Geometry check sheet. Reference: the model listing, model coordinates, mm. Face numbers are marked on the shaded views. A direction names the side the tool comes from. Give positions to 0.01 mm unless a question says otherwise; leave off trailing zeros. Order: outer loops, then holes, each group sorted by start corner. A loop starts at its lowest first (then second) coordinate and runs counter-clockwise, first axis right, second up. Notation, with made-up numbers: M 38.5,82 L 77.5,82 A5 ccw 77.5,86 Z; hole C -7.5,20.5 d11. An arc over 180 degrees is marked long. Answer as CSV lines item,"result".
from build123d import *

# Parameters (mm, degrees)
SKETCH7_R               = 2.5
CUT_EXTRUDE2_DEPTH      = 4
CUT_EXTRUDE3_DEPTH      = 4
CUT_EXTRUDE3_DEPTH_BACK = 4
SKETCH8_W               = 2.5
SKETCH8_H               = 7.259020633
FILLET1_R               = 1.5
SKETCH9_W               = 2.5
SKETCH9_H               = 5.356071321
CUT_EXTRUDE4_DEPTH      = 10
FILLET2_R               = 1.25
SKETCH10_W              = 2.503236591
SKETCH10_H              = 5.356071321
CUT_EXTRUDE5_DEPTH      = 10
SKETCH11_W              = 2.503236591
SKETCH11_H              = 6.001405943
CUT_EXTRUDE6_DEPTH      = 10
FILLET4_R               = 1.25
SKETCH12_W              = 2.514787158
SKETCH12_H              = 5.75
CUT_EXTRUDE9_DEPTH      = 10
SKETCH14_R              = 1.249039751
CUT_EXTRUDE10_DEPTH     = 10


# Some blends are built 0.0001 mm under size
with BuildPart() as part:
    # Sketch5 → Revolve3 (revolve)
    with BuildSketch(Plane.XY, mode=Mode.PRIVATE) as revolve3_sk:
        Polygon((0, 0), (5.5, 0), (5.5, 1), (7, 1), (7, 3), (3, 6), (0, 6), align=None)
    revolve(revolve3_sk.sketch.rotate(Axis((0, 6, 0), (0, -1, 0)), 180), axis=Axis((0, 6, 0), (0, -1, 0)))

    # Sketch7 → Cut-Extrude2 (cut)
    with BuildSketch(Plane(origin=(0, 6, 0), x_dir=(1, 0, 0), z_dir=(0, 1, 0))):
        with Locations(Location((0, 0, 0), (0, 0, 180))):
            Circle(SKETCH7_R)
    extrude(amount=-CUT_EXTRUDE2_DEPTH, mode=Mode.SUBTRACT)

    # Sketch8 → Cut-Extrude3 (cut, two sides: drawn at the far end of the back side and taken through both)
    with BuildSketch(Plane(origin=(0, 2, 0), x_dir=(1, 0, 0), z_dir=(0, 1, 0)).offset(-CUT_EXTRUDE3_DEPTH_BACK)):
        with Locations((0, -3.629510317)):
            Rectangle(SKETCH8_W, SKETCH8_H)
    extrude(amount=CUT_EXTRUDE3_DEPTH + CUT_EXTRUDE3_DEPTH_BACK, mode=Mode.SUBTRACT)

    # Fillet1
    # the kernel refuses this fillet: 1.5 mm, written as the material it adds along each edge
    with BuildSketch(Plane(origin=(1.25, 2, 0), x_dir=(-1, 0, 0), z_dir=(0, -1, 0)), Plane(origin=(-1.25, 0, 0), x_dir=(1, 0, 0), z_dir=(0, 1, 0))) as fillet1_piece_1:
        with BuildLine():
            CenterArc((FILLET1_R, -FILLET1_R), FILLET1_R, 90, 90)
            Line((0, -FILLET1_R), (0, 0))
            Line((0, 0), (FILLET1_R, 0))
        make_face()
    extrude(amount=2)

    # Sketch9 → Cut-Extrude4 (cut)
    with BuildSketch(Plane(origin=(0, 0, 0), x_dir=(-1, 0, 0), z_dir=(0, -1, 0))):
        with Locations((0, -2.67803566)):
            Rectangle(SKETCH9_W, SKETCH9_H)
    extrude(amount=-CUT_EXTRUDE4_DEPTH, mode=Mode.SUBTRACT)

    # Fillet2
    fillet2_edges = [part.edges().sort_by_distance(p)[0] for p in [
        (-1.25, 1, 0),
        (1.25, 1, 0),
    ]]
    fillet(fillet2_edges, radius=FILLET2_R - 0.0001)  # a hair under: the kernel refuses the full size

    # Sketch10 → Cut-Extrude5 (cut)
    with BuildSketch(Plane.XZ):
        with Locations((-0.001618296, 2.67803566)):
            Rectangle(SKETCH10_W, SKETCH10_H)
    extrude(amount=-CUT_EXTRUDE5_DEPTH, mode=Mode.SUBTRACT)

    # Sketch11 → Cut-Extrude6 (cut)
    with BuildSketch(Plane(origin=(0, 0, 0), x_dir=(-1, 0, 0), z_dir=(0, -1, 0))):
        with Locations((0.001618296, -2.355368349)):
            Rectangle(SKETCH11_W, SKETCH11_H)
    extrude(amount=-CUT_EXTRUDE6_DEPTH, mode=Mode.SUBTRACT)

    # Fillet4
    fillet4_edges = [part.edges().sort_by_distance(p)[0] for p in [
        (1.25, 1, -0.645334622),
        (-1.253236591, 1, -0.645334622),
    ]]
    fillet(fillet4_edges, radius=FILLET4_R)

    # Sketch12 → Cut-Extrude9 (cut)
    with BuildSketch(Plane.XZ):
        with Locations((-0.007393579, 2.481071321)):
            Rectangle(SKETCH12_W, SKETCH12_H)
    extrude(amount=-CUT_EXTRUDE9_DEPTH, mode=Mode.SUBTRACT)

    # Sketch14 → Cut-Extrude10 (cut)
    with BuildSketch(Plane(origin=(0, 0, 0), x_dir=(-1, 0, 0), z_dir=(0, -1, 0))):
        with Locations((0.007393579, 0.393928679)):
            Circle(SKETCH14_R)
    extrude(amount=-CUT_EXTRUDE10_DEPTH, mode=Mode.SUBTRACT)


solid = part.part
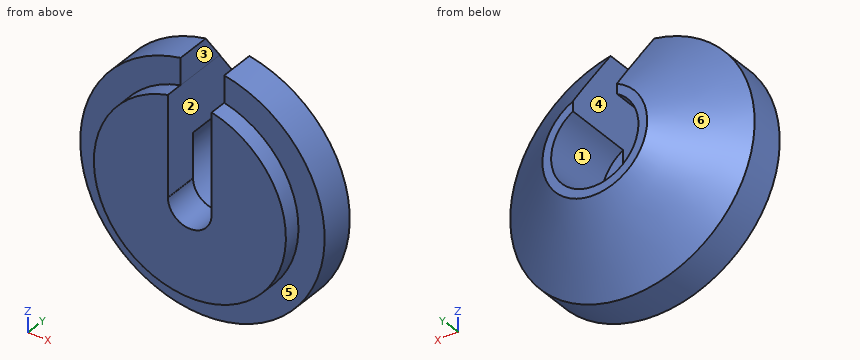
(1) Draft check along X on the marked faces 4, 5 and 6. Enter one of: +X half, -X half, draft (parallel to the pull), parting line (faces both ways), or undercut.
The answers:
face 4,"undercut"
face 5,"draft"
face 6,"parting line"
(2) Gauge pin test, flat ends, axial feed: P1, Ø1.5, axis at x = 4.5, z = 0, coming from the +Y side; P2, Ø1, axis at x = -4.5, z = -0.5, coming from the +Y side; P3, Ø3, axis at x = 0, z = 0, coming from the +Y side. Record the tip position at first contact, or that the pin passes through.
The answers:
P1,"stops at y = 5.44"
P2,"stops at y = 5.23"
P3,"stops at y = 2"
(3) Section check C-C on x = 0. Enter the section's corners in (y, z), then the cut area to 3 significant figures.
The answers:
outline,"M 0,-5.5 L 1,-5.5 L 1,-7 L 3,-7 L 6,-3 L 6,-2.5 L 2,-2.5 L 2,-1.64 L 0,-1.64 Z"
area,"21.2 mm2"
(4) Section check A-A on z = 0. Enter the section's corners in (x, y).
The answers:
outline,"M -7,1 L -5.5,1 L -5.5,0 L -1.26,0 L -1.26,2 L -2.5,2 L -2.5,6 L -3,6 L -7,3 Z; M 1.25,0 L 5.5,0 L 5.5,1 L 7,1 L 7,3 L 3,6 L 2.5,6 L 2.5,2 L 1.25,2 Z"
(5) Tool access check on the marked faces 1, 2 and 3. Record the directions out of +Z, -Z, +X, -X, +Y, -Y that give a thin tool (end or side, any length) a straight path to the whole face; none if there is none.
The answers:
face 1,"+Y"
face 2,"+Y, -Y"
face 3,"+Z, +Y, -Y"
(6) Material ranges on line 1 (X direction, y = 4.75, z = 3.5); line 2 (X direction, y = 4, z = 0); line 3 (Y direction, x = 2, z = -1.25), recorded low to high.
The answers:
line 1,"x = -3.09 to -1.26, 1.25 to 3.09"
line 2,"x = -5.67 to -2.5, 2.5 to 5.67"
line 3,"y = 0 to 2"
